Verification items for this drawing (mm, ordinates from the low corner). A direction names the side the tool comes from. Coordinates: 2 decimals unless noted, no trailing zeros. Write each loop counter-clockwise with the first axis right and the second up, starting at its lowest first coordinate (ties: lowest second). Pieces come first, ordered by that corner, then holes. Notation, with made-up numbers: (13.5, 5.25) -> (42.5, 5.25) arc R18 cw to (42.5, 28.25) -> close; hole circle Ø4 at (65.25, -10). An arc over 180 degrees is marked (long way). Use CSV: the item, a comma, the result in double quotes.
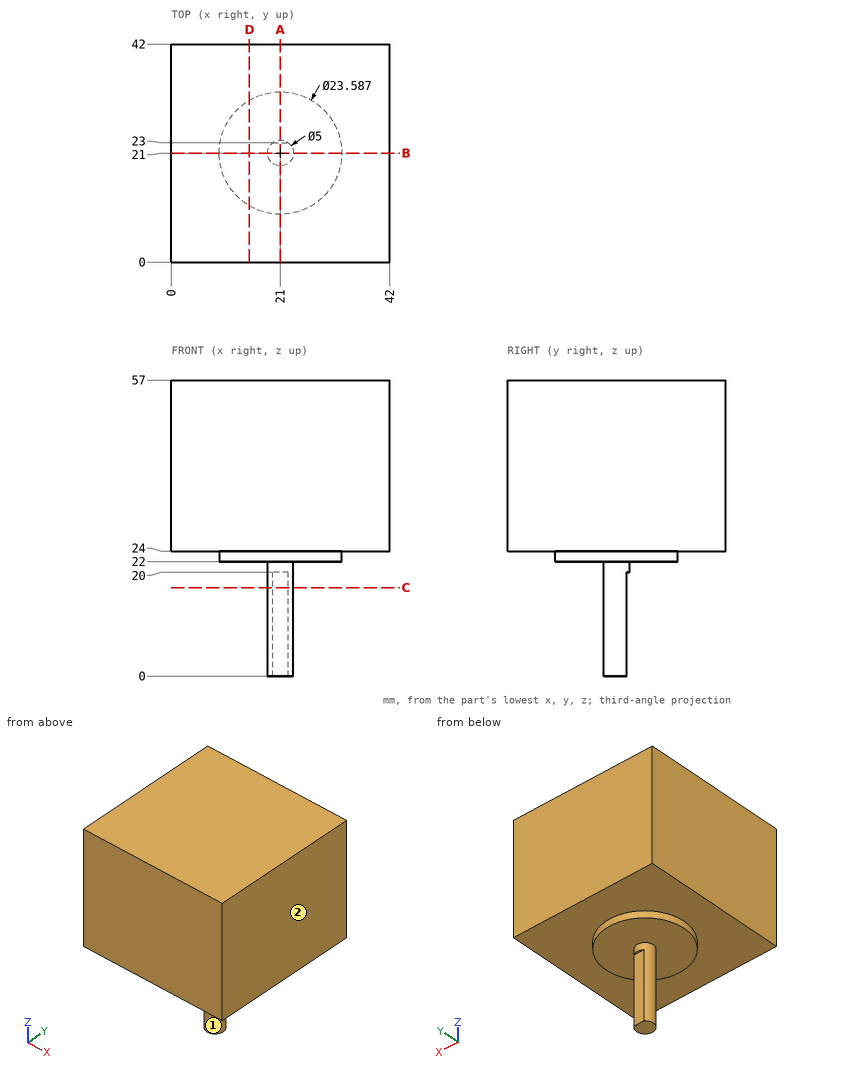
1) Cross-section at C-C (z = 17). Record the boundary of the cut face in (x, y), plus the area to 3 significant figures.
Return value:
outline,"(19.5, 23) arc R2.5 ccw (long way) to (22.5, 23) -> close"
area,"18.6 mm2"
2) Cross-section at A-A (x = 21). Record the boundary of the cut face in (y, z).
Return value:
outline,"(0, 24) -> (9.21, 24) -> (9.21, 22) -> (18.5, 22) -> (18.5, 0) -> (23, 0) -> (23, 20) -> (23.5, 20) -> (23.5, 22) -> (32.79, 22) -> (32.79, 24) -> (42, 24) -> (42, 57) -> (0, 57) -> close"
3) Gauge pin test, flat ends, axial feed: pin 1 (12 mm diameter, centred on x = 30, y = 13.5, fed in from -Z); pin 2 (0.9 mm diameter, centred on x = 21, z = 14.5, fed in from +Y); pin 3 (8 mm diameter, centred on y = 24.5, z = 7, fed in from +X). Record the tip position at first contact, or that the pin passes through.
Return value:
pin 1,"z = 22"
pin 2,"y = 23"
pin 3,"x = 23.5"
4) Cross-section at B-B (y = 21). Record the boundary of the cut face in (x, z), plus the area to 3 significant figures.
Return value:
outline,"(0, 24) -> (9.21, 24) -> (9.21, 22) -> (18.5, 22) -> (18.5, 0) -> (23.5, 0) -> (23.5, 22) -> (32.79, 22) -> (32.79, 24) -> (42, 24) -> (42, 57) -> (0, 57) -> close"
area,"1,540 mm2"
5) Scan lines: L1, parallel to Z at x = 15, y = 27.5; L2, parallel to Z at x = 26, y = 38; L3, parallel to Y at x = 19, z = 4.5. Record each from-to range of solid material in increasing order.
Return value:
L1,"22 to 57"
L2,"24 to 57"
L3,"19.5 to 22.5"
6) Set-up check for the marked faces 1 and 2: record each of +Z, -Z, +X, -X, +Y, -Y from which the full face is reachable in a straight line by a thin tool's end or side.
Return value:
face 1,"-Z"
face 2,"+Z, -Z, +X, +Y, -Y"
7) Cross-section at D-D (x = 15). Record the boundary of the cut face in (y, z).
Return value:
outline,"(0, 24) -> (10.85, 24) -> (10.85, 22) -> (31.15, 22) -> (31.15, 24) -> (42, 24) -> (42, 57) -> (0, 57) -> close"
